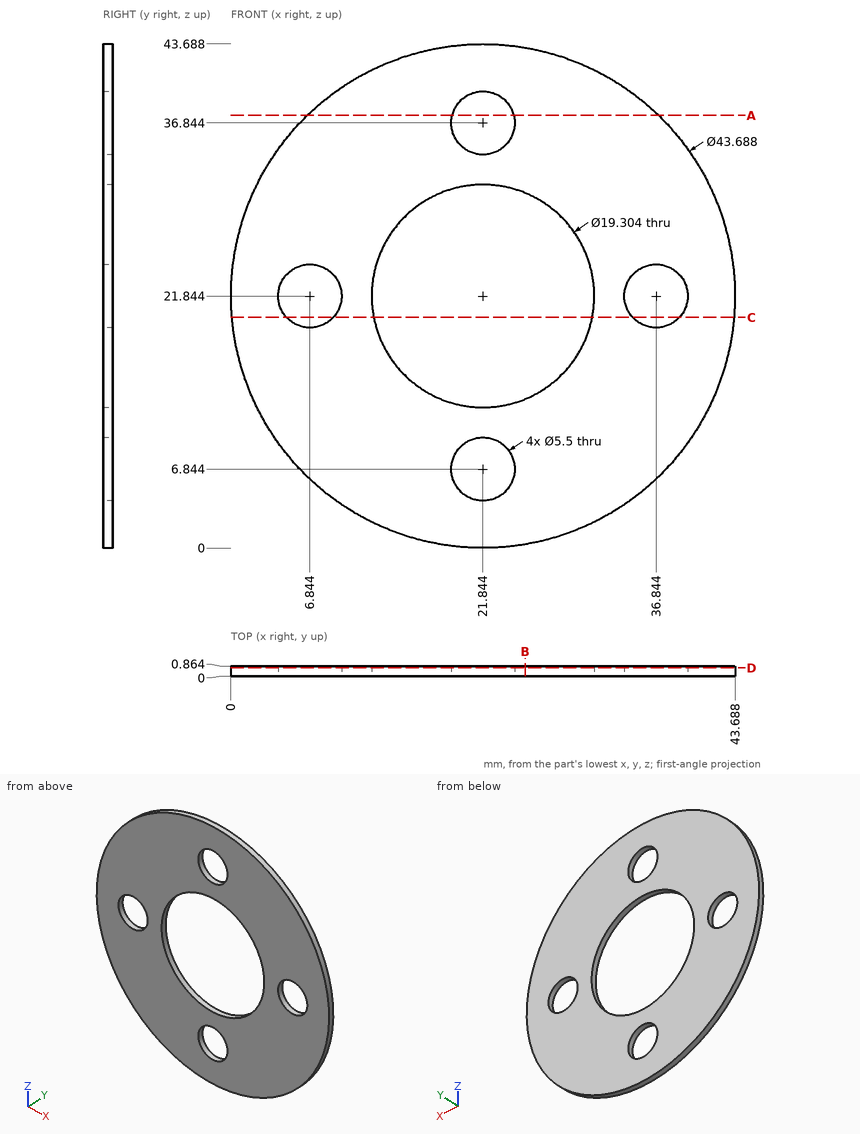
Input: dimensioned drawing with shaded views. Units: mm. Origin: part minimum x, y, z. Coordinates: 2 decimals unless noted, no trailing zeros. Order: outer loops, then holes, each group sorted by start corner. A loop starts at its lowest first (then second) coordinate and runs counter-clockwise, first axis right, second up. Notation, with made-up numbers: (42.5, 81.5) - (96.5, 81.5) arc R18 cw to (96.5, 89.5) - close; hole circle Ø10 at (81.5, 2). An arc over 180 degrees is marked (long way). Return JSON: item names as keys, results as strings. Group by question number.
1. Cut plane C-C (z = 20). Output: boundary loops of the cut face in (x, y), plus the area to 3 significant figures.
2. Cut plane B-B (x = 25.5). Output: boundary loops of the cut face in (y, z).
3. Pin query (flat end, axial travel): pin 1 (3.5 mm diameter, centred on x = 6.844, z = 21.844, fed in from -Y). Return the tip coordinate at first contact, or that it passes through.
4. Cut plane A-A (z = 37.5). Output: boundary loops of the cut face in (x, y) (1 decimal), plus the area to 3 significant figures.
5. Material intervals for line 1 along X through (y, z) = (0.4, 19.5) (1 decimal); line 2 along Z through (x, y) = (21.5, 0.3) (1 decimal); line 3 along Z through (x, y) = (6.5, 0.1) (1 decimal), sorted ascending. Write a range as [from, to].
6. Cut plane D-D (y = 0.7). Output: boundary loops of the cut face in (x, z), plus the area to 3 significant figures.
Resolved:
{
 "1": {"outline": "(0.08, 0) - (4.8, 0) - (4.8, 0.86) - (0.08, 0.86) - close; (8.88, 0) - (12.37, 0) - (12.37, 0.86) - (8.88, 0.86) - close; (31.32, 0) - (34.8, 0) - (34.8, 0.86) - (31.32, 0.86) - close; (38.88, 0) - (43.61, 0) - (43.61, 0.86) - (38.88, 0.86) - close", "area": "14.2 mm²"},
 "2": {"outline": "(0, 0.31) - (0.86, 0.31) - (0.86, 12.91) - (0, 12.91) - close; (0, 30.78) - (0.86, 30.78) - (0.86, 43.38) - (0, 43.38) - close"},
 "3": {"pin 1": "passes through"},
 "4": {"outline": "(6.6, 0) - (19.2, 0) - (19.2, 0.9) - (6.6, 0.9) - close; (24.5, 0) - (37.1, 0) - (37.1, 0.9) - (24.5, 0.9) - close", "area": "21.7 mm²"},
 "5": {"line 1": "x = [0.1, 5.4], [8.3, 12.5], [31.2, 35.4], [38.3, 43.6]", "line 2": "z = [0, 4.1], [9.6, 12.2], [31.5, 34.1], [39.6, 43.7]", "line 3": "z = [6.3, 19.1], [24.6, 37.4]"},
 "6": {"outline": "circle Ø43.69 at (21.84, 21.84); hole circle Ø5.5 at (6.84, 21.84); hole circle Ø19.3 at (21.84, 21.84); hole circle Ø5.5 at (21.84, 6.84); hole circle Ø5.5 at (21.84, 36.84); hole circle Ø5.5 at (36.84, 21.84)", "area": "1,110 mm²"}
}
